Design review of the part built by this model. Coordinates are the model's own, in mm. A direction names the side the tool comes from. Give positions to 0.01 mm unless a question says otherwise; leave off trailing zeros. Loops run counter-clockwise (first coordinate to the right, second up) from the corner with the lowest first, then second, coordinate; pieces in that order, holes last. Notation, with made-up numbers: (-24, -2.75) -> (-19, -2.75) arc R20 ccw to (-19, 36.25) -> close; hole circle Ø6 at (-24, 5). An arc over 180 degrees is marked (long way). Use a Markdown table: item, result. Add a question column.
1. Add section A-A (x = 0). State the section outline as (y, z) points.
2. For pin 1 Ø0.6 at (x, z) = (51, 84.5) entering from -Y; pin 2 Ø24 at (x, z) = (1.5, 73.5) entering from +Y; pin 3 Ø1 at (x, y) = (51, 10.5) entering from -Z, all flat-tipped, find the tip position at first contact; note any pin that passes through.
3. To check wall thickness, follow line 1 (X direction, y = 31.5, z = 113); line 2 (X direction, y = -48, z = 40). State the ranges of each line that lie inside material, in increasing order.
4. Add section C-C (z = 20). State the section outline as (x, y) points.
5. For faces 1 (the cylindrical face through (0, -55, 25)), 2 (the flat face through (-1, 1, 0)), 3 (the cylindrical face through (0, 55, 25)), list the 3-axis set-ups (+Z, -Z, +X, -X, +Y, -Y) from which the entire face can be reached by the end or side of a thin tool; tool diameter is ignored.
6. Add section D-D (x = -32.5). State the section outline as (y, z) points, and give its area (3 significant figures).
7. Add section B-B (z = 91.5). State the section outline as (x, y) points, and give its area (3 significant figures).
```python
from build123d import *

# Parameters (mm, degrees)
SKETCH1_W                = 100
SKETCH1_H                = 100
BOSS_EXTRUDE1_DEPTH      = 150
FILLET1_R                = 10
SKETCH2_W                = 39.23098356
SKETCH2_H                = 63.007337234
BOSS_EXTRUDE2_DEPTH      = 2
BOSS_EXTRUDE3_DEPTH      = 10
BOSS_EXTRUDE3_DEPTH_BACK = 110
SKETCH3_R                = 5


with BuildPart() as part:
    # Sketch1 → Boss-Extrude1 (new body)
    with BuildSketch(Plane.XY):
        Rectangle(SKETCH1_W, SKETCH1_H)
    extrude(amount=BOSS_EXTRUDE1_DEPTH)

    # Fillet1
    fillet1_edges = [part.edges().sort_by_distance(p)[0] for p in [
        (50, -50, 75),
        (-50, -50, 75),
        (-50, 50, 75),
        (50, 50, 75),
    ]]
    fillet(fillet1_edges, radius=FILLET1_R)

    # Sketch2 → Boss-Extrude2 (add)
    with BuildSketch(Plane(origin=(50, 0, 0), x_dir=(0, 0, -1), z_dir=(1, 0, 0))):
        with Locations((-75, 0)):
            Rectangle(SKETCH2_W, SKETCH2_H)
    extrude(amount=BOSS_EXTRUDE2_DEPTH)

    # Sketch3 → Boss-Extrude3 (add, two sides: drawn at the far end of the back side and taken through both)
    with BuildSketch(Plane.XZ.offset(50).offset(-BOSS_EXTRUDE3_DEPTH_BACK)):
        with Locations(Location((0, 20, 0), (0, 0, 270))):
            Circle(SKETCH3_R)
    extrude(amount=BOSS_EXTRUDE3_DEPTH + BOSS_EXTRUDE3_DEPTH_BACK)


solid = part.part
```
Taken from the geometry:
| question | item | result |
|---|---|---|
| 1 | outline | (-60, 15) -> (-50, 15) -> (-50, 0) -> (50, 0) -> (50, 15) -> (60, 15) -> (60, 25) -> (50, 25) -> (50, 150) -> (-50, 150) -> (-50, 25) -> (-60, 25) -> close |
| 2 | pin 1 | stops at y = -31.5 |
| 2 | pin 2 | stops at y = 50 |
| 2 | pin 3 | stops at z = 55.38 |
| 3 | line 1 | x = -50 to 50 |
| 3 | line 2 | x = -46 to 46 |
| 4 | outline | (-50, -40) arc R10 ccw to (-40, -50) -> (-5, -50) -> (-5, -60) -> (5, -60) -> (5, -50) -> (40, -50) arc R10 ccw to (50, -40) -> (50, 40) arc R10 ccw to (40, 50) -> (5, 50) -> (5, 60) -> (-5, 60) -> (-5, 50) -> (-40, 50) arc R10 ccw to (-50, 40) -> close |
| 5 | face 1 | -Y |
| 5 | face 2 | -Z, +X, -X, +Y, -Y |
| 5 | face 3 | +Y |
| 6 | outline | (-50, 0) -> (50, 0) -> (50, 150) -> (-50, 150) -> close |
| 6 | area | 15,000 mm^2 |
| 7 | outline | (-50, -40) arc R10 ccw to (-40, -50) -> (40, -50) arc R10 ccw to (50, -40) -> (50, -31.5) -> (52, -31.5) -> (52, 31.5) -> (50, 31.5) -> (50, 40) arc R10 ccw to (40, 50) -> (-40, 50) arc R10 ccw to (-50, 40) -> close |
| 7 | area | 10,000 mm^2 |
